Verification items for the finished model (mm, model axes). Face numbers are marked on the shaded views. A direction names the side the tool comes from. Round coordinates to 2 decimals unless told otherwise and drop trailing zeros. Order: outer loops, then holes, each group sorted by start corner. A loop starts at its lowest first (then second) coordinate and runs counter-clockwise, first axis right, second up. Notation, with made-up numbers: (61, -25.5) -> (109, -25.5) arc R6 cw to (109, -21.5) -> close; hole circle Ø7 at (56.25, 77.5). An arc over 180 degrees is marked (long way). Write item = value, one per line. Start each with the question number.
from build123d import *

# Parameters (mm, degrees)
F0_W           = 55
F0_H           = 40
F12_DEPTH      = 50
F1_W           = 35
F1_H           = 40
F13_DEPTH      = 40.001
F14_T1_DEPTH   = 111.7855168217
F14_T3_DEPTH   = 111.7855168217
F15_R          = 2
F2_DEPTH       = 55.001
F3_R           = 7.5
F3_R_2         = 2
F16_DEPTH      = 3
F6_D           = 3
F6_CSINK_D     = 7
F6_CSINK_ANGLE = 90
F7_R           = 2
F8_DEPTH       = 5
F17_R          = 4
F17_R_2        = 2
F9_DEPTH       = 5


# Not quite as in the source:
# - a fillet or chamfer that OpenCascade refuses, or shapes differently, is made with other operations: its cross-section is extruded or revolved along the edge and cut away or added


with BuildPart() as f12:
    # F0 (on Top) → F12 (new body)
    with BuildSketch(Plane.XY):
        Rectangle(F0_W, F0_H)
    extrude(amount=F12_DEPTH)

    # F1 (on face) → F13 (cut, through all)
    with BuildSketch(Plane.XZ.offset(20)):
        with Locations((0, 30)):
            Rectangle(F1_W, F1_H)
    extrude(amount=-F13_DEPTH, mode=Mode.SUBTRACT)

    # F14: fillet of radius 20.3571033643 on 4 edges, made by hand

    # F14_s2 → F14_t1 (cut)
    with BuildSketch(Plane.YZ.offset(-33.3927584109)):
        with BuildLine():
            ThreePointArc((-20, 29.6428966357), (-14.0375424699, 44.0375424699), (0.3571033643, 50))
            Line((0.3571033643, 50), (-20, 50))
            Line((-20, 50), (-20, 29.6428966357))
        make_face()
        with BuildLine():
            ThreePointArc((-0.3571033643, 50), (14.0375424699, 44.0375424699), (20, 29.6428966357))
            Line((20, 29.6428966357), (20, 50))
            Line((20, 50), (-0.3571033643, 50))
        make_face()
    extrude(amount=F14_T1_DEPTH, mode=Mode.SUBTRACT)

    # F14_s4 → F14_t3 (cut)
    with BuildSketch(Plane.YZ.offset(-78.3927584109)):
        with BuildLine():
            ThreePointArc((-20, 29.6428966357), (-14.0375424699, 44.0375424699), (0.3571033643, 50))
            Line((0.3571033643, 50), (-20, 50))
            Line((-20, 50), (-20, 29.6428966357))
        make_face()
        with BuildLine():
            ThreePointArc((-0.3571033643, 50), (14.0375424699, 44.0375424699), (20, 29.6428966357))
            Line((20, 29.6428966357), (20, 50))
            Line((20, 50), (-0.3571033643, 50))
        make_face()
    extrude(amount=F14_T3_DEPTH, mode=Mode.SUBTRACT)

    # F15 (on face) → F2 (cut, through all)
    with BuildSketch(Plane.YZ.offset(27.5)):
        with Locations((0, 29.6428966357)):
            Circle(F15_R)
    extrude(amount=-F2_DEPTH, mode=Mode.SUBTRACT)

    # F3 (on face) → F16 (join)
    with BuildSketch(Plane.YZ.offset(-17.5)):
        with Locations((0, 29.6428966357)):
            Circle(F3_R)
        with Locations((0, 29.6428966357)):
            Circle(F3_R_2, mode=Mode.SUBTRACT)
    extrude(amount=F16_DEPTH)

    # F4: F12 across plane


with BuildPart() as f12_1:
    add(f12.part)
    add(f12.part.mirror(Plane.YZ))

    # F6 (through all)
    with Locations(Plane.XY.offset(10)):
        with Locations((0, 12), (0, -12)):
            CounterSinkHole(F6_D / 2, F6_CSINK_D / 2, counter_sink_angle=F6_CSINK_ANGLE)

    # F7 (on face) → F8 (cut)
    with BuildSketch(Plane.YZ.offset(27.5)):
        Polygon((0.4025775089, 25.6017005954), (3.8796188691, 27.6616803799), (3.8341447246, 31.7028764202), (0.3116292198, 33.6840926759), (-3.1654121404, 31.6241128914), (-3.1199379959, 27.5829168512), align=None)
        with Locations((0, 29.6428966357)):
            Circle(F7_R, mode=Mode.SUBTRACT)
    extrude(amount=-F8_DEPTH, mode=Mode.SUBTRACT)

    # F17 (on face) → F9 (cut)
    with BuildSketch(Plane(origin=(-27.5, 0, 0), x_dir=(0, -1, 0), z_dir=(-1, 0, 0))):
        with Locations((0, 29.6428966357)):
            Circle(F17_R)
        with Locations((0, 29.6428966357)):
            Circle(F17_R_2, mode=Mode.SUBTRACT)
    extrude(amount=-F9_DEPTH, mode=Mode.SUBTRACT)


solid = f12_1.part
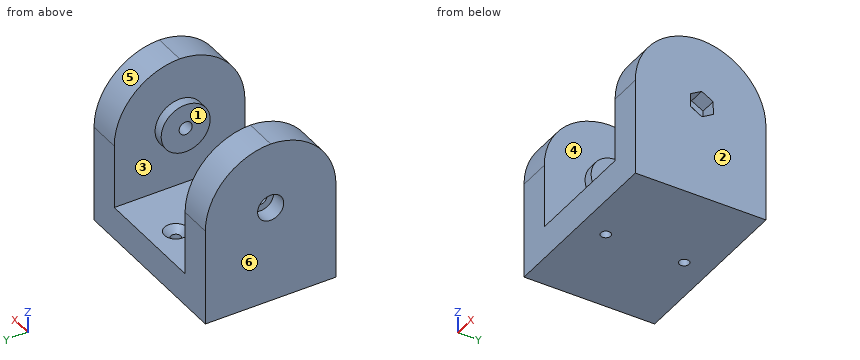
(1) Cross-section at C-C (y = -12). Enter the section's corners in (x, z).
(2) Cross-section at B-B (x = 0). Enter the section's corners in (y, z).
(3) Draft check along Z on the marked faces 3, 4, 5 and 6. Enter one of: +Z half, -Z half, draft (parallel to the pull), parting line (faces both ways), or undercut.
(4) Scan lines: line 1 along Y through (x, z) = (0, 5.75); line 2 along Z through (x, y) = (-24.15, 0); line 3 along X through (y, z) = (1, 41). Record each from-to range of solid material in increasing order. Write a range as from..to.
(5) Cross-section at A-A (z = 15). Enter the section's corners in (x, y), and give its area (3 significant figures).
(6) Cross-section at D-D (x = -18.5). Enter the section's corners in (y, z).
(7) Depth check by flat-ended pin: pin 1 (7.5 mm diameter, centred on y = -0.5, z = 27, fed in from -X); pin 2 (17.5 mm diameter, centred on x = -4.5, y = 5.5, fed in from +Z); pin 3 (4 mm diameter, centred on y = 0, z = 31, fed in from -X). Enter the tip coordinate at first touch or a pass-through.
(8) Set-up check for the marked faces 1 and 2: record each of +Z, -Z, +X, -X, +Y, -Y from which the full face is reachable in a straight line by a thin tool's end or side.
Outcome:
q1.outline = (-27.5, 0) -> (-1.5, 0) -> (-1.5, 8) -> (-3.5, 10) -> (-17.5, 10) -> (-17.5, 45.82) -> (-27.5, 45.82) -> close; (1.5, 0) -> (27.5, 0) -> (27.5, 45.82) -> (17.5, 45.82) -> (17.5, 10) -> (3.5, 10) -> (1.5, 8) -> close
q2.outline = (-20, 0) -> (-13.5, 0) -> (-13.5, 8) -> (-15.5, 10) -> (-20, 10) -> close; (-10.5, 0) -> (10.5, 0) -> (10.5, 8) -> (8.5, 10) -> (-8.5, 10) -> (-10.5, 8) -> close; (13.5, 0) -> (20, 0) -> (20, 10) -> (15.5, 10) -> (13.5, 8) -> close
q3.face_3 = undercut
q3.face_4 = undercut
q3.face_5 = +Z half
q3.face_6 = draft
q4.line_1 = -20..-13.5, -10.5..10.5, 13.5..20
q4.line_2 = 0..25.64, 33.64..50
q4.line_3 = -27.5..-17.5, 17.5..27.5
q5.outline = (-27.5, -20) -> (-17.5, -20) -> (-17.5, 20) -> (-27.5, 20) -> close; (17.5, -20) -> (27.5, -20) -> (27.5, 20) -> (17.5, 20) -> close
q5.area = 800 mm^2
q6.outline = (-20, 0) -> (20, 0) -> (20, 29.64) arc R20.36 ccw to (0, 50) arc R20.36 ccw to (-20, 29.64) -> close; hole circle Ø4 at (0, 29.64)
q7.pin_1 = -27.5
q7.pin_2 = 10
q7.pin_3 = -22.5
q8.face_1 = +Z, +Y, -Y
q8.face_2 = +Z, -Z, +X, +Y, -Y
